The model under review builds one solid part; all positions refer to its coordinate system, in mm. Face numbers are marked on the shaded views. A direction names the side the tool comes from. Round coordinates to 2 decimals unless told otherwise and drop trailing zeros. Write each loop counter-clockwise with the first axis right and the second up, starting at its lowest first coordinate (ties: lowest second). Pieces come first, ordered by that corner, then holes. Notation, with made-up numbers: (66, -20.5) - (97, -20.5) arc R29 ccw to (97, 5.5) - close; hole circle Ø2 at (-7, 47.25). An arc over 180 degrees is marked (long way). Write each question's results on one line, items separated by ' | '.
```python
from build123d import *

# Parameters (mm, degrees)
SKETCH_R      = 2
SKETCH_R_2    = 1.5
SKETCH_R_3    = 5.75
PAD_DEPTH     = 4
PAD001_DEPTH  = 10
SKETCH002_R   = 3
SKETCH002_R_2 = 2.5
POCKET_DEPTH  = 2
FILLET_R      = 1


with BuildPart() as part:
    # Sketch → Pad (new body)
    with BuildSketch(Plane.XY):
        with BuildLine():
            ThreePointArc((-45, 25), (-48.535534, 23.535534), (-50, 20))
            Line((-50, -20), (-50, 20))
            ThreePointArc((-50, -20), (-48.535534, -23.535534), (-45, -25))
            Line((45, -25), (-45, -25))
            ThreePointArc((45, -25), (48.535534, -23.535534), (50, -20))
            Line((50, 20), (50, -20))
            ThreePointArc((50, 20), (48.535534, 23.535534), (45, 25))
            Line((-45, 25), (45, 25))
        make_face()
        with Locations((-45, 20)):
            Circle(SKETCH_R, mode=Mode.SUBTRACT)
        with Locations((45, 20)):
            Circle(SKETCH_R, mode=Mode.SUBTRACT)
        with Locations((-45, -20)):
            Circle(SKETCH_R, mode=Mode.SUBTRACT)
        with Locations((45, -20)):
            Circle(SKETCH_R, mode=Mode.SUBTRACT)
        with Locations((-31, 3)):
            Circle(SKETCH_R_2, mode=Mode.SUBTRACT)
        with Locations((0, 3)):
            Circle(SKETCH_R_2, mode=Mode.SUBTRACT)
        with Locations((22, 3)):
            Circle(SKETCH_R_3, mode=Mode.SUBTRACT)
        with BuildLine():
            ThreePointArc((-23, 7.5), (-23.707107, 7.207107), (-24, 6.5))
            Line((-24, -0.5), (-24, 6.5))
            ThreePointArc((-24, -0.5), (-23.707107, -1.207107), (-23, -1.5))
            Line((-8, -1.5), (-23, -1.5))
            ThreePointArc((-8, -1.5), (-7.292893, -1.207107), (-7, -0.5))
            Line((-7, 6.5), (-7, -0.5))
            ThreePointArc((-7, 6.5), (-7.292893, 7.207107), (-8, 7.5))
            Line((-23, 7.5), (-8, 7.5))
        make_face(mode=Mode.SUBTRACT)
    extrude(amount=-PAD_DEPTH)

    # Sketch001 (on Face25 of Pad) → Pad001 (join)
    with BuildSketch(Plane(origin=(0, 0, -4), x_dir=(1, 0, 0), z_dir=(0, 0, -1))):
        with BuildLine():
            ThreePointArc((-30, 15), (-37.071068, 12.071068), (-40, 5))
            Line((-40, -5), (-40, 5))
            ThreePointArc((-40, -5), (-37.071068, -12.071068), (-30, -15))
            Line((30, -15), (-30, -15))
            ThreePointArc((30, -15), (37.071068, -12.071068), (40, -5))
            Line((40, 5), (40, -5))
            ThreePointArc((40, 5), (37.071068, 12.071068), (30, 15))
            Line((-30, 15), (30, 15))
        make_face()
        with BuildLine():
            ThreePointArc((-30, 13), (-35.656854, 10.656854), (-38, 5))
            Line((-38, -5), (-38, 5))
            ThreePointArc((-38, -5), (-35.656854, -10.656854), (-30, -13))
            Line((30, -13), (-30, -13))
            ThreePointArc((30, -13), (35.656854, -10.656854), (38, -5))
            Line((38, 5), (38, -5))
            ThreePointArc((38, 5), (35.656854, 10.656854), (30, 13))
            Line((-30, 13), (30, 13))
        make_face(mode=Mode.SUBTRACT)
    extrude(amount=PAD001_DEPTH)

    # Sketch002 (on Face4 of Pad001) → Pocket (cut)
    with BuildSketch(Plane.XY):
        with Locations((-45, 20)):
            Circle(SKETCH002_R)
        with Locations((45, 20)):
            Circle(SKETCH002_R)
        with Locations((45, -20)):
            Circle(SKETCH002_R)
        with Locations((-45, -20)):
            Circle(SKETCH002_R)
        with Locations((-31, 3)):
            Circle(SKETCH002_R_2)
        with Locations((0, 3)):
            Circle(SKETCH002_R_2)
    extrude(amount=-POCKET_DEPTH, mode=Mode.SUBTRACT)

    # Fillet
    fillet_edges = [part.edges().sort_by_distance(p)[0] for p in [
        (0, -25, 0),
    ]]
    fillet(fillet_edges, radius=FILLET_R)


solid = part.part
```
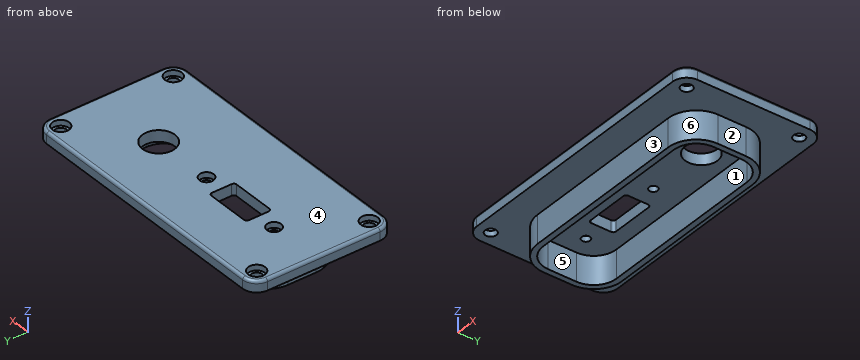
Q1. For probe 1 along Y at (x, z) = (-45, -2.5); probe 2 along Y at (x, z) = (-3, -8); probe 3 along Y at (x, z) = (0, -3.3), list the stretches that pass through material, from the lowest coordinate up.
Evaluation:
probe 1: y = -25 to -22, -18 to 18, 22 to 25 | probe 2: y = -15 to -13, 13 to 15 | probe 3: y = -25 to 1.5, 4.5 to 25
Q2. We need section C-C (y = 3). State how many separate pieces and enclosed holes the cut face has, plus the area to 3 significant figures.
Evaluation:
separate pieces: 5 | enclosed holes: 0 | area: 294 mm^2
Q3. We need section B-B (x = 0). State the section outline as (y, z) points, plus the area to 3 significant figures.
Evaluation:
outline: (-25, -4) - (-15, -4) - (-15, -14) - (-13, -14) - (-13, -4) - (1.5, -4) - (1.5, -2) - (0.5, -2) - (0.5, 0) - (-24, 0) arc R1 ccw to (-25, -1) - close; (4.5, -4) - (13, -4) - (13, -14) - (15, -14) - (15, -4) - (25, -4) - (25, -1) arc R1 ccw to (24, 0) - (5.5, 0) - (5.5, -2) - (4.5, -2) - close | area: 224 mm^2
Q4. Insertion check: P1, Ø3, axis at x = -45.5, y = 19.5, coming from the +Z side; P2, Ø10, axis at x = -0.5, y = -18, coming from the -Z side; P3, Ø4.5, axis at x = 45, y = -20, coming from the -Z side; P4, Ø5, axis at y = -4, z = -8, coming from the +X side. Each pin has a flat end and moves straight along its axis. Give the tip position at first contact, or say it passes through.
Evaluation:
P1: stops at z = -2 | P2: stops at z = -14 | P3: stops at z = -4 | P4: stops at x = 40
Q5. We need section A-A (z = -9). State the section outline as (x, y) points, plus the area to 3 significant figures.
Evaluation:
outline: (-40, -5) arc R10 ccw to (-30, -15) - (30, -15) arc R10 ccw to (40, -5) - (40, 5) arc R10 ccw to (30, 15) - (-30, 15) arc R10 ccw to (-40, 5) - close; hole (-38, -5) arc R8 ccw to (-30, -13) - (30, -13) arc R8 ccw to (38, -5) - (38, 5) arc R8 ccw to (30, 13) - (-30, 13) arc R8 ccw to (-38, 5) - close | area: 393 mm^2
Q6. Tool access review of the marked faces 1, 2 and 3: name each direction out of +Z, -Z, +X, -X, +Y, -Y from which nothing blocks a thin tool from reaching the whole face with its end or side.
Evaluation:
face 1: -Z | face 2: -Z, +X, +Y, -Y | face 3: -Z, +X, -X, -Y
Q7. We need section D-D (x = 37). State the section outline as (y, z) points.
Evaluation:
outline: (-25, -4) - (-12.14, -4) - (-12.14, -14) - (-8.87, -14) - (-8.87, -4) - (8.87, -4) - (8.87, -14) - (12.14, -14) - (12.14, -4) - (25, -4) - (25, -1) arc R1 ccw to (24, 0) - (-24, 0) arc R1 ccw to (-25, -1) - close
Q8. The part is to be moulded in two halves that separate along Y. For the marked faces 4, 5 and 6, say which applies: released by +Y, released by -Y, zero draft, split by the parting line, or undercut.
Evaluation:
face 4: zero draft | face 5: undercut | face 6: released by -Y
